from build123d import *

# Parameters (mm, degrees)
SKETCH_2_W             = 28
SKETCH_2_H             = 4.5
CUT_EXTRUDE_1_DEPTH    = 10
EXTRUDE_1_DEPTH        = 15
HOLE_WIZARD_M3_1_D     = 2.5
HOLE_WIZARD_M3_1_DEPTH = 4
HOLE_WIZARD_M3_1_TIP   = 0.751075774
CUT_EXTRUDE_START      = -20
CUT_EXTRUDE_2_DEPTH    = 20
HOLE_WIZARD_M4_1_D     = 3.3
HOLE_WIZARD_M4_1_DEPTH = 10.1
HOLE_WIZARD_M4_1_TIP   = 0.991420021
HOLE_WIZARD_M3_2_D     = 2.5
HOLE_WIZARD_M5_1_D     = 4.2
HOLE_WIZARD_M5_1_DEPTH = 14
HOLE_WIZARD_M5_1_TIP   = 1.2618073
SCALE_1_SCALE          = 0.8
SCALE_2_SCALE          = 0.8
SCALE_3_SCALE          = 0.8


with BuildPart() as part:
    # 草图1 → 旋转1 (revolve)
    with BuildSketch(Plane.XY, mode=Mode.PRIVATE) as revolve_1_sk:
        Polygon((0, 0), (4.1, 0), (4.1, 6.7), (13.4, 6.7), (13.4, 8.7), (21, 8.7), (21, 10.2), (20, 10.2), (20, 11.2), (21, 11.2), (21, 12.2), (10, 12.2), (10, 13.2), (21, 13.2), (21, 20.4), (5, 20.4), (5, 21), (21, 21), (21, 34.7), (18.3, 38.7), (3.5, 38.7), (3.5, 43.7), (0, 43.7), align=None)
    revolve(revolve_1_sk.sketch.rotate(Axis((0, 43.7, 0), (0, -1, 0)), 90), axis=Axis((0, 43.7, 0), (0, -1, 0)))

    # 草图2 → 切除-拉伸1 (cut)
    with BuildSketch(Plane.XY.offset(21)):
        with Locations((0, 16.05)):
            Rectangle(SKETCH_2_W, SKETCH_2_H)
    extrude(amount=-CUT_EXTRUDE_1_DEPTH, mode=Mode.SUBTRACT)

    # 草图3 → 凸台-拉伸1 (add)
    with BuildSketch(Plane.XY.offset(11)):
        with BuildLine():
            Line((9.185056323, 18.053194417), (9.385056323, 18.053194417))
            ThreePointArc((9.385056323, 18.053194417), (11.385056323, 16.053194417), (9.385056323, 14.053194417))
            Line((9.385056323, 14.053194417), (9.185056323, 14.053194417))
            ThreePointArc((9.185056323, 14.053194417), (7.185056323, 16.053194417), (9.185056323, 18.053194417))
        make_face()
    extrude(amount=EXTRUDE_1_DEPTH)

    # M3 螺纹孔1
    with Locations(Plane(origin=(0, 38.7, 0), x_dir=(1, 0, 0), z_dir=(0, 1, 0))):
        with Locations((-6.5, 0), (6.5, 0)):
            Hole(HOLE_WIZARD_M3_1_D / 2, depth=HOLE_WIZARD_M3_1_DEPTH)
            with Locations((0, 0, -(HOLE_WIZARD_M3_1_DEPTH + HOLE_WIZARD_M3_1_TIP / 2))):  # 118° drill point
                Cone(0, HOLE_WIZARD_M3_1_D / 2, HOLE_WIZARD_M3_1_TIP, mode=Mode.SUBTRACT)

    # 草图7 → 旋转2 (revolve)
    with BuildSketch(Plane.XY, mode=Mode.PRIVATE) as revolve_2_sk:
        Polygon((0, -54.6), (5, -54.6), (5, -30.5), (8.275, -30.5), (8.275, -29.6), (13, -29.6), (13, -27.6), (21, -27.6), (21, 8.7), (0, 8.7), align=None)
    revolve(revolve_2_sk.sketch.rotate(Axis((0, 8.7, 0), (0, -1, 0)), 180), axis=Axis((0, 8.7, 0), (0, -1, 0)))

    # 草图8 → 切除-拉伸2 (cut)
    with BuildSketch(Plane.XZ.offset(54.6).offset(CUT_EXTRUDE_START)):
        with BuildLine():
            Line((-3, 4), (3, 4))
            ThreePointArc((3, 4), (0, 5), (-3, 4))
        make_face()
    extrude(amount=CUT_EXTRUDE_2_DEPTH, mode=Mode.SUBTRACT)

    # M4 螺纹孔1
    with Locations(Plane(origin=(0, -27.6, 0), x_dir=(-1, 0, 0), z_dir=(0, -1, 0))):
        with Locations((17.5, 0), (0, -17.5), (-17.5, 0), (0, 17.5)):
            Hole(HOLE_WIZARD_M4_1_D / 2, depth=HOLE_WIZARD_M4_1_DEPTH)
            with Locations((0, 0, -(HOLE_WIZARD_M4_1_DEPTH + HOLE_WIZARD_M4_1_TIP / 2))):  # 118° drill point
                Cone(0, HOLE_WIZARD_M4_1_D / 2, HOLE_WIZARD_M4_1_TIP, mode=Mode.SUBTRACT)

    # M3 螺纹孔2 (through all)
    with Locations(Plane(origin=(0, -44.6, 4), x_dir=(1, 0, 0), z_dir=(0, 0, 1))):
        with Locations((0, 0)):
            Hole(HOLE_WIZARD_M3_2_D / 2)

    # M5 螺纹孔1
    with Locations(Plane(origin=(0, -54.6, 0), x_dir=(-1, 0, 0), z_dir=(0, -1, 0))):
        with Locations((0, 0)):
            Hole(HOLE_WIZARD_M5_1_D / 2, depth=HOLE_WIZARD_M5_1_DEPTH)
            with Locations((0, 0, -(HOLE_WIZARD_M5_1_DEPTH + HOLE_WIZARD_M5_1_TIP / 2))):  # 118° drill point
                Cone(0, HOLE_WIZARD_M5_1_D / 2, HOLE_WIZARD_M5_1_TIP, mode=Mode.SUBTRACT)


with BuildPart() as part_1:
    # 缩放比例1: scaled about (0, 0, 0)
    add(part.part.scale(SCALE_1_SCALE))


with BuildPart() as part_2:
    # 缩放比例2: scaled about (0, 0, 0)
    add(part_1.part.scale(SCALE_2_SCALE))


with BuildPart() as part_3:
    # 缩放比例3: scaled about (0, 0, 0)
    add(part_2.part.scale(SCALE_3_SCALE))


solid = part_3.part
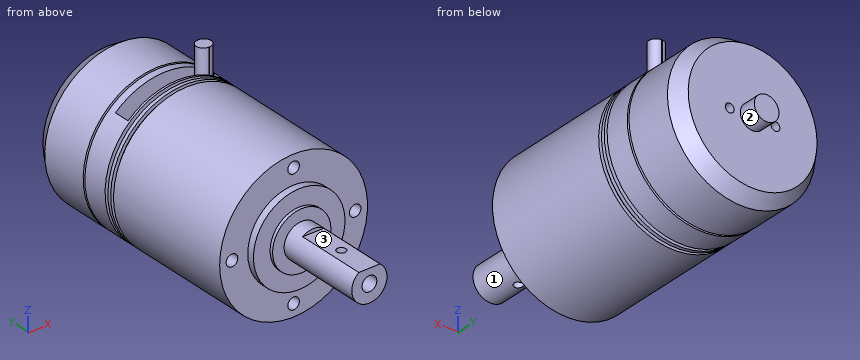
The model under review builds one solid part; all positions refer to its coordinate system, in mm. Face numbers are marked on the shaded views. A direction names the side the tool comes from. Give positions to 0.01 mm unless a question says otherwise; leave off trailing zeros. Loops run counter-clockwise (first coordinate to the right, second up) from the corner with the lowest first, then second, coordinate; pieces in that order, holes last. Notation, with made-up numbers: (64.25, -30) -> (101.25, -30) arc R20 ccw to (101.25, -16) -> close; hole circle Ø10 at (6, 87.5). An arc over 180 degrees is marked (long way). Put each result on its own line as item: value. Start each with the question number.
1. Wall thickness on probe 1 along Y at (x, z) = (-5, -7.25); probe 2 along Y at (x, z) = (-3, -5); probe 3 along Y at (x, z) = (-1.75, 6.75): over which ranges is each line inside the solid? List them lowest first.
2. For the marked faces 1, 2 and 3, list the 3-axis set-ups (+Z, -Z, +X, -X, +Y, -Y) from which the entire face can be reached by the end or side of a thin tool; tool diameter is ignored.
3. We need section B-B on z = 11.75. State the section outline as (x, y) points, then the cut area to 3 significant figures.
4. We need section D-D on y = -18.5. State the section outline as (x, z) points, then the cut area to 3 significant figures.
5. Clearance check with flat-ended pins moving along their axes: P1, Ø1.5, axis at x = -8.96, z = 0, coming from the +Y side; P2, Ø1.5, axis at y = -8, z = 7, coming from the -X side; P3, Ø3, axis at y = 3.5, z = -7.5, coming from the +X side. State where each tip first meets the part, or that it passes through.
6. We need section A-A on y = -3. State the section outline as (x, z) points.
7. We need section C-C on y = 18.5. State the section outline as (x, z) points, then the cut area to 3 significant figures.
Determined:
1. probe 1: -14.13 to 6.25, 6.76 to 10.44, 10.75 to 19.81
1. probe 2: -15.16 to 6.25, 6.76 to 10.44, 10.75 to 19.81
1. probe 3: -14.13 to 6.25, 6.76 to 7.07, 9.37 to 10.44, 10.75 to 19.81
2. face 1: -Y
2. face 2: +Y
2. face 3: +Z, +X, -X, -Y
3. outline: (4.7, 7.2) -> (4.81, 7.2) arc R1.02 ccw to (4.81, 9.24) -> (4.7, 9.24) arc R1.02 ccw to start
3. area: 3.50 mm^2
4. outline: (-1.54, 2.05) arc R2.56 ccw (long way) to (1.54, 2.05) -> close
4. area: 19.5 mm^2
5. P1: y = 19.81
5. P2: x = -8.75
5. P3: x = 8.92
6. outline: circle Ø21.5 at (0, 0)
7. outline: circle Ø20.51 at (0, 0); hole circle Ø1.28 at (-3.33, 0); hole circle Ø1.28 at (3.33, 0)
7. area: 328 mm^2
